The drawing under review shows one solid part. Ordinate dimensions are in mm from its lowest x, y, z. Round coordinates to 2 decimals unless told otherwise and drop trailing zeros. Order: outer loops, then holes, each group sorted by start corner. A loop starts at its lowest first (then second) coordinate and runs counter-clockwise, first axis right, second up. Notation, with made-up numbers: (-9.5, 3) -> (49.5, 3) arc R19 ccw to (49.5, 24) -> close; hole circle Ø3 at (5.5, -10). An arc over 180 degrees is marked (long way). Use a Markdown table: item, result. Add a question column.
1) Consider section B-B (x = 10.5). State the section outline as (y, z) points.
2) Consider section D-D (x = 20). State the section outline as (y, z) points, plus the area to 3 significant figures.
3) Consider section A-A (y = 47.5). State the section outline as (x, z) points, plus the area to 3 significant figures.
4) Consider section C-C (z = 0.6). State the section outline as (x, y) points.
5) Clearance check with a flat-ended pin moving along its axis: P1, Ø4, axis at x = 20, y = 87.5, coming from the -Z side. State where the tip first meets the part, or that it passes through.
6) Wall thickness on line 1 along Y through (x, z) = (20, 0.95); line 2 along Y through (x, z) = (10.5, 1); line 3 along X through (y, z) = (8.5, 1.25): over which ranges is each line inside the solid? List them lowest first. Write a range as [from, to].
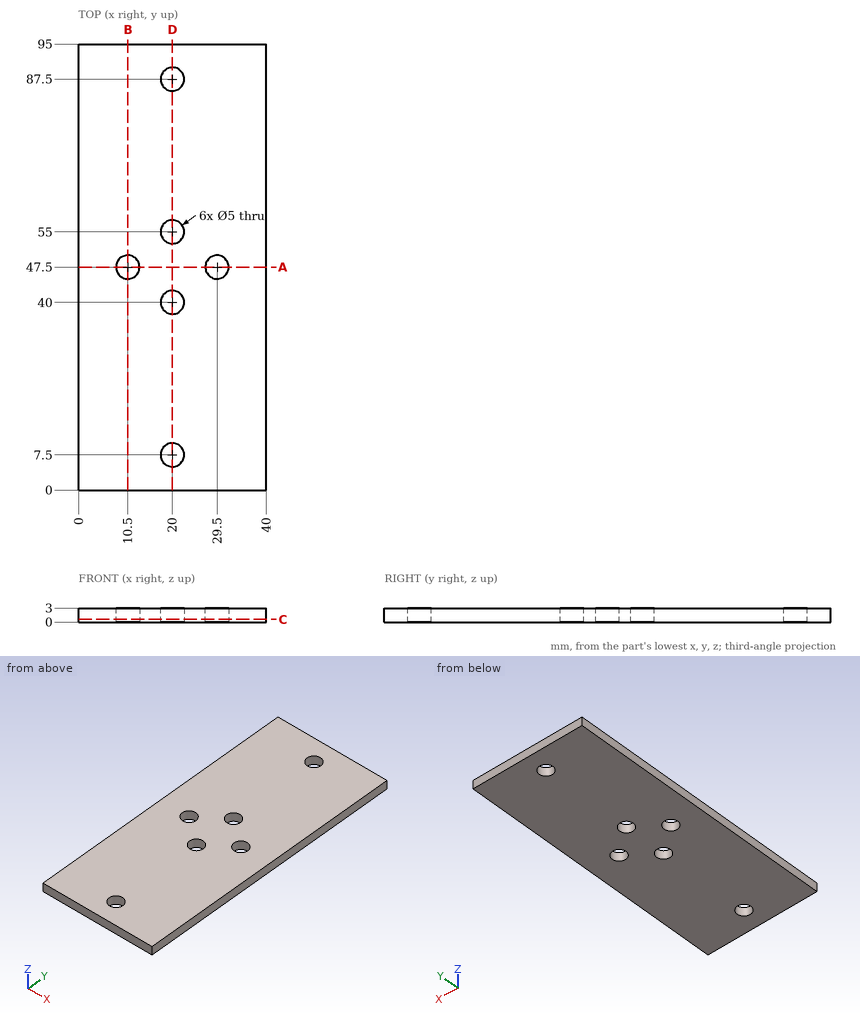
Results list:
| question | item | result |
|---|---|---|
| 1 | outline | (0, 0) -> (45, 0) -> (45, 3) -> (0, 3) -> close; (50, 0) -> (95, 0) -> (95, 3) -> (50, 3) -> close |
| 2 | outline | (0, 0) -> (5, 0) -> (5, 3) -> (0, 3) -> close; (10, 0) -> (37.5, 0) -> (37.5, 3) -> (10, 3) -> close; (42.5, 0) -> (52.5, 0) -> (52.5, 3) -> (42.5, 3) -> close; (57.5, 0) -> (85, 0) -> (85, 3) -> (57.5, 3) -> close; (90, 0) -> (95, 0) -> (95, 3) -> (90, 3) -> close |
| 2 | area | 225 mm2 |
| 3 | outline | (0, 0) -> (8, 0) -> (8, 3) -> (0, 3) -> close; (13, 0) -> (27, 0) -> (27, 3) -> (13, 3) -> close; (32, 0) -> (40, 0) -> (40, 3) -> (32, 3) -> close |
| 3 | area | 90.0 mm2 |
| 4 | outline | (0, 0) -> (40, 0) -> (40, 95) -> (0, 95) -> close; hole circle Ø5 at (10.5, 47.5); hole circle Ø5 at (20, 7.5); hole circle Ø5 at (20, 40); hole circle Ø5 at (20, 55); hole circle Ø5 at (20, 87.5); hole circle Ø5 at (29.5, 47.5) |
| 5 | P1 | through |
| 6 | line 1 | [0, 5], [10, 37.5], [42.5, 52.5], [57.5, 85], [90, 95] |
| 6 | line 2 | [0, 45], [50, 95] |
| 6 | line 3 | [0, 17.71], [22.29, 40] |
